from build123d import *

# Parameters (mm, degrees)
M4_TAPPED_HOLE1_D     = 3.3
M4_TAPPED_HOLE1_DEPTH = 10.508579979
M4_TAPPED_HOLE1_TIP   = 0.991420021


with BuildPart() as part:
    # Sketch1 → Revolve1 (revolve)
    with BuildSketch(Plane.XY, mode=Mode.PRIVATE) as revolve1_sk:
        Polygon((0, 0), (15, 0), (15, 7), (10, 9), (10, 17), (6, 17), (6, 5), (0, 5), align=None)
    revolve(revolve1_sk.sketch.rotate(Axis((0, 5, 0), (0, -1, 0)), 180), axis=Axis((0, 5, 0), (0, -1, 0)))

    # M4 Tapped Hole1
    with Locations(Plane(origin=(0, 0, 0), x_dir=(-1, 0, 0), z_dir=(0, -1, 0))):
        with Locations((0, 0)):
            Hole(M4_TAPPED_HOLE1_D / 2, depth=M4_TAPPED_HOLE1_DEPTH)
            with Locations((0, 0, -(M4_TAPPED_HOLE1_DEPTH + M4_TAPPED_HOLE1_TIP / 2))):  # 118° drill point
                Cone(0, M4_TAPPED_HOLE1_D / 2, M4_TAPPED_HOLE1_TIP, mode=Mode.SUBTRACT)


solid = part.part
For this review, take the finished solid that the model builds, in its own axes (mm). A direction names the side the tool comes from. Give positions to 0.01 mm unless a question says otherwise; leave off trailing zeros. Order: outer loops, then holes, each group sorted by start corner. A loop starts at its lowest first (then second) coordinate and runs counter-clockwise, first axis right, second up. Notation, with made-up numbers: M 30,84.5 L 73,84.5 A3 cw 73,89.5 Z; hole C 81,-28 d9. An arc over 180 degrees is marked long. Answer in a Markdown table with one row per item. Add a question column.
(1) Consider section A-A on z = 0. State the section outline as (x, y) points, and give its area (4 significant figures).
(2) Consider section B-B on x = 0. State the section outline as (y, z) points.
(3) For faces 1 (the face through (10, 13, 0)), 2 (the face through (-1.216, 2.535, -1.115)), list the 3-axis set-ups (+Z, -Z, +X, -X, +Y, -Y) from which the entire face can be reached by the end or side of a thin tool; tool diameter is ignored.
(4) Wall thickness on probe 1 along Z at (x, y) = (0, 14.75); probe 2 along Y at (x, z) = (-3, -4.5); probe 3 along Z at (x, y) = (0, 1.6): over which ranges is each line inside the solid? List them lowest first. Write a range as [from, to].
(5) Consider section C-C on y = 9.75. State the section outline as (x, z) points, and give its area (3 significant figures).
(6) Mouldability with a two-part tool opening along X and no side actions: class faces 3 (the face through (-7, 17, 0)), 4 (the face through (-1.2, 5, -1.4)), 5 (the face through (-8.06, 3.55, -12.65)) as +X half, -X half, draft (parallel to the pull), parting line (faces both ways), or undercut.
(7) For pin 1 (3 mm diameter, centred on x = -11, y = 4, fed in from +Z); pin 2 (1 mm diameter, centred on x = 0, y = 13, fed in from +Z); pin 3 (10 mm diameter, centred on y = 9.5, z = -6.5, fed in from -X), all flat-tipped, find the tip position at first contact; note any pin that passes through.
Evaluation:
| question | item | result |
|---|---|---|
| 1 | outline | M -15,0 L -1.65,0 L -1.65,5 L -6,5 L -6,17 L -10,17 L -10,9 L -15,7 Z; M 1.65,0 L 15,0 L 15,7 L 10,9 L 10,17 L 6,17 L 6,5 L 1.65,5 Z |
| 1 | area | 259.5 mm^2 |
| 2 | outline | M 0,-15 L 7,-15 L 9,-10 L 17,-10 L 17,-6 L 5,-6 L 5,-1.65 L 0,-1.65 Z; M 0,1.65 L 5,1.65 L 5,6 L 17,6 L 17,10 L 9,10 L 7,15 L 0,15 Z |
| 3 | face 1 | +Y |
| 3 | face 2 | +Y, -Y |
| 4 | probe 1 | z = [-10, -6], [6, 10] |
| 4 | probe 2 | y = [0, 5] |
| 4 | probe 3 | z = [-15, -1.65], [1.65, 15] |
| 5 | outline | C 0,0 d20; hole C 0,0 d12 |
| 5 | area | 201 mm^2 |
| 6 | face 3 | draft |
| 6 | face 4 | undercut |
| 6 | face 5 | parting line |
| 7 | pin 1 | stops at z = 11.61 |
| 7 | pin 2 | stops at z = 10 |
| 7 | pin 3 | stops at x = -14.84 |
